from build123d import *

# Parameters (mm, degrees)
SKETCH1_W           = 30
SKETCH1_H           = 30
BOSS_EXTRUDE1_DEPTH = 25
SKETCH3_W           = 10
SKETCH3_H           = 10
CUT_EXTRUDE1_DEPTH  = 20
SKETCH4_R           = 8
CUT_EXTRUDE2_DEPTH  = 15
SKETCH5_W           = 20
SKETCH5_H           = 20
BOSS_EXTRUDE2_DEPTH = 5
SKETCH6_W           = 10
SKETCH6_H           = 10
CUT_EXTRUDE3_DEPTH  = 15


with BuildPart() as part:
    # Sketch1 → Boss-Extrude1 (new body)
    with BuildSketch(Plane(origin=(0, 0, 0), x_dir=(1, 0, 0), z_dir=(0, 1, 0))):
        with Locations((15, 15)):
            Rectangle(SKETCH1_W, SKETCH1_H)
    extrude(amount=BOSS_EXTRUDE1_DEPTH)

    # Sketch3 → Cut-Extrude1 (cut)
    with BuildSketch(Plane(origin=(0, 25, 0), x_dir=(1, 0, 0), z_dir=(0, 1, 0))):
        with Locations((15, 15)):
            Rectangle(SKETCH3_W, SKETCH3_H)
    extrude(amount=-CUT_EXTRUDE1_DEPTH, mode=Mode.SUBTRACT)

    # Sketch4 → Cut-Extrude2 (cut)
    with BuildSketch(Plane.ZY):
        with Locations((-15, 10)):
            Circle(SKETCH4_R)
    extrude(amount=-CUT_EXTRUDE2_DEPTH, mode=Mode.SUBTRACT)

    # Sketch5 → Boss-Extrude2 (add)
    with BuildSketch(Plane(origin=(0, 25, 0), x_dir=(1, 0, 0), z_dir=(0, 1, 0))):
        with Locations((15, 15)):
            Rectangle(SKETCH5_W, SKETCH5_H)
    extrude(amount=BOSS_EXTRUDE2_DEPTH)

    # Sketch6 → Cut-Extrude3 (cut)
    with BuildSketch(Plane(origin=(0, 30, 0), x_dir=(1, 0, 0), z_dir=(0, 1, 0))):
        with Locations((15, 15)):
            Rectangle(SKETCH6_W, SKETCH6_H)
    extrude(amount=-CUT_EXTRUDE3_DEPTH, mode=Mode.SUBTRACT)


solid = part.part
Here's how the part is built. I have some questions about the finished solid (model axes, mm). A direction names the side the tool comes from. Give positions to 0.01 mm unless a question says otherwise; leave off trailing zeros. Order: outer loops, then holes, each group sorted by start corner. A loop starts at its lowest first (then second) coordinate and runs counter-clockwise, first axis right, second up. Notation, with made-up numbers: (-2, 68) -> (18, 68) arc R15 cw to (18, 73) -> close; hole circle Ø9 at (14.5, 29.25). An arc over 180 degrees is marked (long way). One line per item, written item: value. Start each with the question number.
1. Imagine slicing it at C-C, the plane x = 18.75. List the corners of the cut face in (y, z) for me.
2. I need wall thicknesses on probe 1 along Z at (x, y) = (6.75, 10); probe 2 along Z at (x, y) = (17.25, 28); probe 3 along Y at (x, z) = (4, -15). Which ranges of each line are inside material? Lowest first, please. Write a range as from..to.
3. We'd pull the mould along X, two halves only. Please class faces 1 (the face through (16, 20, -20)), 2 (the face through (17, 5, -15)), 3 (the face through (10, 23, -15)), 4 (the face through (15, 4, -15)): released by +X, released by -X, zero draft, split by the parting line, or undercut.
4. Will these pins go through, and if not, where does the flat tip stop? pin 1 Ø5.5 at (x, z) = (17, -15.5) entering from +Y; pin 2 Ø4.5 at (y, z) = (8.5, -18) entering from -X; pin 3 Ø2.5 at (x, y) = (10.5, 28.5) entering from -Z.
5. Imagine slicing it at A-A, the plane z = -15. List the corners of the cut face in (x, y) for me.
6. For faces 5 (the face through (25, 27, -15)), 6 (the face through (15, 27, -5)), 7 (the face through (5, 27, -15)), 8 (the face through (16, 20, -10)), which set-ups out of +Z, -Z, +X, -X, +Y, -Y let a thin tool reach every point of the face, with its end or its side?
7. Imagine slicing it at B-B, the plane y = 25.5. List the corners of the cut face in (x, z) for me.
8. Imagine slicing it at D-D, the plane z = -24.25. List the corners of the cut face in (x, y) for me.
Values follow:
1. outline: (0, -30) -> (25, -30) -> (25, -25) -> (30, -25) -> (30, -20) -> (5, -20) -> (5, -10) -> (30, -10) -> (30, -5) -> (25, -5) -> (25, 0) -> (0, 0) -> close
2. probe 1: z = -30..-23, -7..0
2. probe 2: z = -25..-20, -10..-5
2. probe 3: y = 0..2, 18..25
3. face 1: undercut
3. face 2: zero draft
3. face 3: undercut
3. face 4: released by -X
4. pin 1: stops at y = 5
4. pin 2: stops at x = 15
4. pin 3: stops at z = -25
5. outline: (0, 0) -> (30, 0) -> (30, 25) -> (25, 25) -> (25, 30) -> (20, 30) -> (20, 5) -> (15, 5) -> (15, 2) -> (0, 2) -> close; (0, 18) -> (10, 18) -> (10, 30) -> (5, 30) -> (5, 25) -> (0, 25) -> close
6. face 5: +Z, -Z, +X, +Y
6. face 6: +Z, +X, -X, +Y
6. face 7: +Z, -Z, -X, +Y
6. face 8: +Y
7. outline: (5, -25) -> (25, -25) -> (25, -5) -> (5, -5) -> close; hole (10, -20) -> (20, -20) -> (20, -10) -> (10, -10) -> close
8. outline: (0, 0) -> (30, 0) -> (30, 25) -> (25, 25) -> (25, 30) -> (5, 30) -> (5, 25) -> (0, 25) -> close
